```python
from build123d import *

# Parameters (mm, degrees)
SKETCH1_W                       = 55.372
SKETCH1_H                       = 21.59
BOSS_EXTRUDE1_DEPTH             = 4.1599866
SKETCH2_W                       = 4.064
SKETCH2_H                       = 21.59
BOSS_EXTRUDE2_DEPTH             = 39.0200134
M3_CLEARANCE_HOLE2_D            = 3.4
SKETCH1_2_W                     = 55.372
SKETCH1_2_H                     = 21.59
BOSS_EXTRUDE3_DEPTH             = 2.54
CBORE_FOR_M5_SBHCS1_D           = 5.5
CBORE_FOR_M5_SBHCS1_CBORE_D     = 10.5
CBORE_FOR_M5_SBHCS1_CBORE_DEPTH = 2.75
FILLET1_R                       = 0.762


with BuildPart() as part:
    # Sketch1 → Boss-Extrude1 (new body)
    with BuildSketch(Plane(origin=(0, 0, 0), x_dir=(1, 0, 0), z_dir=(0, 1, 0))):
        with Locations((27.686, 10.795)):
            Rectangle(SKETCH1_W, SKETCH1_H)
    extrude(amount=BOSS_EXTRUDE1_DEPTH)

    # Sketch2 → Boss-Extrude2 (add)
    with BuildSketch(Plane(origin=(0, 4.1599866, 0), x_dir=(1, 0, 0), z_dir=(0, 1, 0))):
        with Locations((2.032, 10.795)):
            Rectangle(SKETCH2_W, SKETCH2_H)
        with Locations((53.34, 10.795)):
            Rectangle(SKETCH2_W, SKETCH2_H)
    extrude(amount=BOSS_EXTRUDE2_DEPTH)

    # M3 Clearance Hole2 (through all)
    with Locations(Plane.ZY):
        with Locations((-10.795, 37.8599954), (-10.795, 12.4599954)):
            Hole(M3_CLEARANCE_HOLE2_D / 2)

    # Sketch1<2> → Boss-Extrude3 (add)
    with BuildSketch(Plane(origin=(0, 0, 0), x_dir=(1, 0, 0), z_dir=(0, 1, 0))):
        with Locations((27.686, 10.795)):
            Rectangle(SKETCH1_2_W, SKETCH1_2_H)
    extrude(amount=-BOSS_EXTRUDE3_DEPTH)

    # CBORE for M5 SBHCS1 (through all)
    with Locations(Plane(origin=(0, 4.1599866, 0), x_dir=(1, 0, 0), z_dir=(0, 1, 0))):
        with Locations((11.811, 10.795), (43.561, 10.795)):
            CounterBoreHole(CBORE_FOR_M5_SBHCS1_D / 2, CBORE_FOR_M5_SBHCS1_CBORE_D / 2, CBORE_FOR_M5_SBHCS1_CBORE_DEPTH)

    # Fillet1
    fillet1_edges = [part.edges().sort_by_distance(p)[0] for p in [
        (27.686, 4.1599866, 0),
        (4.064, 23.6699933, 0),
        (4.064, 23.6699933, -21.59),
        (0, 43.18, -10.795),
        (4.064, 43.18, -10.795),
        (27.686, 4.1599866, -21.59),
        (51.308, 23.6699933, -21.59),
        (51.308, 23.6699933, 0),
        (55.372, 43.18, -10.795),
        (51.308, 43.18, -10.795),
        (0, 20.32, -21.59),
        (55.372, 20.32, -21.59),
        (55.372, 20.32, 0),
        (0, 20.32, 0),
    ]]
    fillet(fillet1_edges, radius=FILLET1_R)


solid = part.part
```
Input: part model. Units: mm. Frame: model coordinates. A direction names the side the tool comes from. Round coordinates to 2 decimals unless told otherwise and drop trailing zeros. Order: outer loops, then holes, each group sorted by start corner. A loop starts at its lowest first (then second) coordinate and runs counter-clockwise, first axis right, second up. Notation, with made-up numbers: (-20, 6.25) - (-12, 6.25) arc R21 ccw to (-12, 23.25) - close; hole circle Ø4 at (-12.5, 31.5). An arc over 180 degrees is marked (long way). One line per question, with ' | ' between items. Start each with the question number.
1) Cut plane C-C, the plane z = -18. Return the cut outline in (x, y), then the cut area to 3 significant figures.
2) Cut plane B-B, the plane x = 45.5. Return the cut outline in (y, z), then the cut area to 3 significant figures.
3) Pull-direction query (Y, two-part tool) for faces 4 (the flat face through (27, -2.54, -11)), 5 (the cylindrical face through (2.06, 39.546, -10.574)), 6 (the flat face through (46, 1.41, -9)), 7 (the flat face through (32, 2, 0)); classes: +Y half, -Y half, draft (parallel to the pull), parting line (faces both ways), or undercut.
4) Cut plane D-D, the plane x = 26. Return the cut outline in (y, z), then the cut area to 3 significant figures.
5) Cut plane A-A, the plane y = 32. Return the cut outline in (x, z), then the cut area to 3 significant figures.
6) Contact query for flat-ended pins moving along their axis: P1, Ø5, axis at x = 12.5, z = -8, coming from the +Y side; P2, Ø2.5, axis at y = 12.46, z = -10.8, coming from the -X side; P3, Ø6.5, axis at x = 43.561, z = -10.795, coming from the +Y side. Output: stop coordinate, or through.
7) Set-up query: faces 1 (the cylindrical face through (48.41, 2.8, -8.78)), 2 (the flat face through (51.308, 23, -11)), 3 (the cylindrical face through (53.37, 10.95, -11.58)). Return all of +Z, -Z, +X, -X, +Y, -Y with unobstructed straight access to the full face (end or side cutting, diameter ignored); none if empty.
8) Ray query, probe 1 along Y at (x, z) = (2, -11); probe 2 along X at (y, z) = (17, -9); probe 3 along Y at (x, z) = (16.5, -10.25). Return the intervals inside material, ascending.
Worked out:
1) outline: (0, -2.54) - (55.37, -2.54) - (55.37, 42.42) arc R0.76 ccw to (54.61, 43.18) - (52.07, 43.18) arc R0.76 ccw to (51.31, 42.42) - (51.31, 4.16) - (4.06, 4.16) - (4.06, 42.42) arc R0.76 ccw to (3.3, 43.18) - (0.76, 43.18) arc R0.76 ccw to (0, 42.42) - close | area: 688 mm^2
2) outline: (-2.54, -21.59) - (3.4, -21.59) arc R0.76 ccw to (4.16, -20.83) - (4.16, -15.67) - (1.41, -15.67) - (1.41, -12.75) - (-2.54, -12.75) - close; (-2.54, -8.84) - (1.41, -8.84) - (1.41, -5.92) - (4.16, -5.92) - (4.16, -0.76) arc R0.76 ccw to (3.4, 0) - (-2.54, 0) - close | area: 102 mm^2
3) face 4: -Y half | face 5: undercut | face 6: +Y half | face 7: draft
4) outline: (-2.54, -21.59) - (3.4, -21.59) arc R0.76 ccw to (4.16, -20.83) - (4.16, -0.76) arc R0.76 ccw to (3.4, 0) - (-2.54, 0) - close | area: 144 mm^2
5) outline: (0, -20.83) arc R0.76 ccw to (0.76, -21.59) - (3.3, -21.59) arc R0.76 ccw to (4.06, -20.83) - (4.06, -0.76) arc R0.76 ccw to (3.3, 0) - (0.76, 0) arc R0.76 ccw to (0, -0.76) - close; (51.31, -20.83) arc R0.76 ccw to (52.07, -21.59) - (54.61, -21.59) arc R0.76 ccw to (55.37, -20.83) - (55.37, -0.76) arc R0.76 ccw to (54.61, 0) - (52.07, 0) arc R0.76 ccw to (51.31, -0.76) - close | area: 174 mm^2
6) P1: stops at y = 4.16 | P2: passes through | P3: stops at y = 1.41
7) face 1: +Y | face 2: +Z, -Z, +Y | face 3: +X, -X
8) probe 1: y = -2.54 to 10.77, 14.15 to 36.17, 39.55 to 43.18 | probe 2: x = 0 to 4.06, 51.31 to 55.37 | probe 3: y = -2.54 to 1.41
